Here's how the part is built. I have some questions about the finished solid (model axes, mm). Coordinates: 2 decimals unless noted, no trailing zeros. Write each loop counter-clockwise with the first axis right and the second up, starting at its lowest first coordinate (ties: lowest second). Pieces come first, ordered by that corner, then holes. Notation, with made-up numbers: (45.5, -16.75) - (100.5, -16.75) arc R29 cw to (100.5, 18.25) - close; hole circle Ø1 at (-26.5, 28). An arc over 180 degrees is marked (long way). Answer in a Markdown table with one row per item. Add a question column.
Item 1: Imagine slicing it at A-A (x = -122.5). Please give me the cut outline in (y, z), plus the area to 3 significant figures.
Item 2: If I drill on probe 1 along Z at (x, y) = (-55, -17.5); probe 2 along X at (y, z) = (-5.25, 214); probe 3 along Y at (x, z) = (109, -438.6), over which ranges is the centre line in solid material (lowest first)? Write a range as from..to.
Item 3: I'm going to push flat-ended pins straight in: pin 1 (6 mm diameter, centred on y = -12.5, z = 8.5, fed in from -X); pin 2 (7.5 mm diameter, centred on y = -12.5, z = 8.5, fed in from +X). Where does each tip first touch, or does it pass through?
Item 4: Imagine slicing it at B-B (z = -392.5). Please give me the cut outline in (x, y).
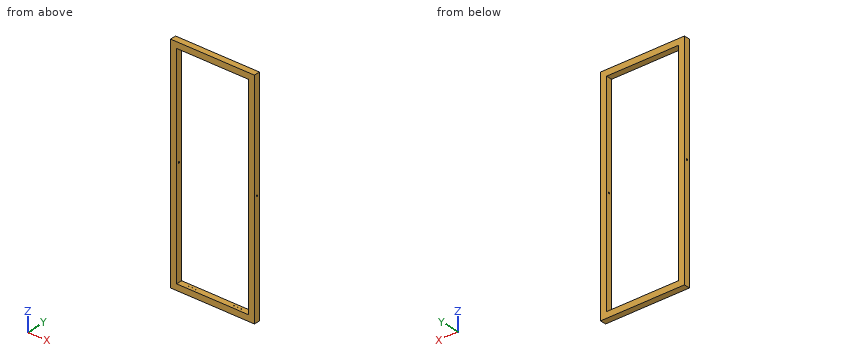
from build123d import *

# Parameters (mm, degrees)
F0_W     = 348
F0_H     = 925
F0_W_2   = 298
F0_H_2   = 875
F1_DEPTH = 25
F3_D     = 6.6
F3_DEPTH = 500
F3_TIP   = 1.9828400428
F4_R     = 1.65
F5_DEPTH = 4
F7_W     = 344.8
F7_H     = 921.8
F7_W_2   = 301.2
F7_H_2   = 878.2
F8_DEPTH = 21.8


with BuildPart() as f1:
    # F0 (on Front) → F1 (new body)
    with BuildSketch(Plane.XZ):
        Rectangle(F0_W, F0_H)
        Rectangle(F0_W_2, F0_H_2, mode=Mode.SUBTRACT)
    extrude(amount=F1_DEPTH)

    # F3
    with Locations(Plane.YZ.offset(174)):
        with Locations((-12.5, 8.5)):
            Hole(F3_D / 2, depth=F3_DEPTH)
            with Locations((0, 0, -(F3_DEPTH + F3_TIP / 2))):  # 118° drill point
                Cone(0, F3_D / 2, F3_TIP, mode=Mode.SUBTRACT)

    # F4 (on face) → F5 (cut)
    with BuildSketch(Plane.XY.offset(-437.5)):
        with Locations((109, -12.5)):
            Circle(F4_R)
        with Locations((94, -12.5)):
            Circle(F4_R)
        with Locations((79, -12.5)):
            Circle(F4_R)
        with Locations((-79, -12.5)):
            Circle(F4_R)
        with Locations((-94, -12.5)):
            Circle(F4_R)
        with Locations((-109, -12.5)):
            Circle(F4_R)
    extrude(amount=-F5_DEPTH, mode=Mode.SUBTRACT)

    # F7 (on offset) → F8 (cut)
    with BuildSketch(Plane.XZ.offset(23.4)):
        Rectangle(F7_W, F7_H)
        Rectangle(F7_W_2, F7_H_2, mode=Mode.SUBTRACT)
    extrude(amount=-F8_DEPTH, mode=Mode.SUBTRACT)


solid = f1.part
Here are the results:
| question | item | result |
|---|---|---|
| 1 | outline | (-25, -462.5) - (0, -462.5) - (0, -437.5) - (-25, -437.5) - close; (-25, 437.5) - (0, 437.5) - (0, 462.5) - (-25, 462.5) - close; hole (-23.4, -460.9) - (-1.6, -460.9) - (-1.6, -439.1) - (-23.4, -439.1) - close; hole (-23.4, 439.1) - (-1.6, 439.1) - (-1.6, 460.9) - (-23.4, 460.9) - close |
| 1 | area | 300 mm2 |
| 2 | probe 1 | z = -462.5..-460.9, -439.1..-437.5, 437.5..439.1, 460.9..462.5 |
| 2 | probe 2 | x = -174..-172.4, -150.6..-149, 149..150.6, 172.4..174 |
| 2 | probe 3 | y = -25..-14.15, -10.85..0 |
| 3 | pin 1 | passes through |
| 3 | pin 2 | stops at x = 174 |
| 4 | outline | (-174, -25) - (-149, -25) - (-149, 0) - (-174, 0) - close; (149, -25) - (174, -25) - (174, 0) - (149, 0) - close; hole (-172.4, -23.4) - (-150.6, -23.4) - (-150.6, -1.6) - (-172.4, -1.6) - close; hole (150.6, -23.4) - (172.4, -23.4) - (172.4, -1.6) - (150.6, -1.6) - close |
